```python
from build123d import *

# Parameters (mm, degrees)
F0_W           = 92.075
F0_H           = 12.7
F1_DEPTH       = 46.0375
F2_R           = 16.8275
F3_DEPTH       = 11.1125
F4_D           = 5.5
F5_R           = 35
F5_R_2         = 16.8275
F6_DEPTH       = 25.4
F7_D           = 12.7
F7_CBORE_D     = 12.7
F7_CBORE_DEPTH = 6.35


# Not quite as in the source:
# - a length typed as a fraction of an inch, garbled in the dataset ("3 / 203.2 mm" for 3/8 in), is restored


with BuildPart() as f1:
    # F0 (on Front) → F1 (new body, symmetric)
    with BuildSketch(Plane.XZ):
        with Locations((7.9375, 6.35)):
            Rectangle(F0_W, F0_H)
    extrude(amount=F1_DEPTH, both=True)

    # F2 (on face) → F3 (cut)
    with BuildSketch(Plane.XY.offset(12.7)):
        Circle(F2_R)
    extrude(amount=-F3_DEPTH, mode=Mode.SUBTRACT)

    # F4 (through all)
    with Locations(Plane.XY.offset(12.7)):
        with Locations((0, 22.5), (22.5, 0), (0, -22.5), (-22.5, 0)):
            Hole(F4_D / 2)

    # F5 (on face) → F6 (intersect)
    with BuildSketch(Plane.XY.offset(12.7)):
        Circle(F5_R)
        Circle(F5_R_2, mode=Mode.SUBTRACT)
        Circle(F5_R_2)
    extrude(amount=-F6_DEPTH, mode=Mode.INTERSECT)

    # F7 (through all)
    with Locations(Plane.XY.offset(12.7)):
        with Locations((0, 0)):
            CounterBoreHole(F7_D / 2, F7_CBORE_D / 2, F7_CBORE_DEPTH)


solid = f1.part
```
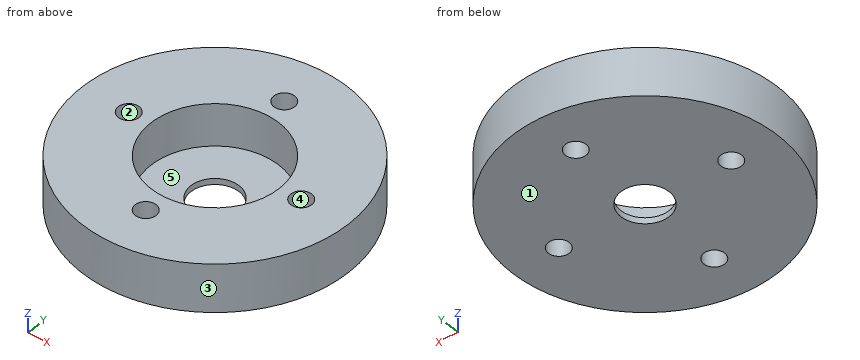
Could you check a few things on this model? Use its own coordinates, in mm. Face numbers are marked on the shaded views. A direction names the side the tool comes from. Round coordinates to 2 decimals unless told otherwise and drop trailing zeros. Write each loop counter-clockwise with the first axis right and the second up, starting at its lowest first coordinate (ties: lowest second). Pieces come first, ordered by that corner, then holes. Notation, with made-up numbers: M 55,25 L 66,25 A23 ccw 66,51 Z; hole C -29.75,34 d1. An arc over 180 degrees is marked long. Answer in a Markdown table with one row per item. Add a question column.
Q1. If I drill on line 1 (Y direction, x = 0, z = 8); line 2 (X direction, y = -2, z = 12.25); line 3 (Y direction, x = -24, z = 3), over which ranges is the centre line in solid material (lowest first)? Write a range as from..to.
Q2. Imagine slicing it at D-D (x = 22.5). Please give me the cut outline in (y, z).
Q3. Imagine slicing it at C-C (z = 4.5). Give the number of separate pieces and of enclosed holes in the cut face, then the cut area to 3 significant figures.
Q4. Will these pins go through, and if not, where does the flat tip stop? pin 1 Ø6 at (x, z) = (-7.5, 6.5) entering from -Y; pin 2 Ø17 at (x, y) = (-3.5, 4) entering from +Z; pin 3 Ø7.5 at (x, y) = (0, 0) entering from +Z; pin 4 Ø6 at (x, z) = (-24.5, 4) entering from -Y.
Q5. If we mould it in two halves opening along Y, with no side actions, what happens to the marked faces 1, 2 and 3? For each: +Y half, -Y half, draft (parallel to the pull), parting line (faces both ways), or undercut.
Q6. On a 3-axis mill with a long thin cutter (end or side, diameter ignored), from which of +Z, -Z, +X, -X, +Y, -Y can I reach the whole of each face in a straight line? I mean the marked faces 4 and 5. Say none if no direction works.
Q7. Imagine slicing it at A-A (x = 0). Please give me the cut outline in (y, z), then the cut area to 3 significant figures.
Values:
| question | item | result |
|---|---|---|
| 1 | line 1 | -35..-25.25, -19.75..-16.83, 16.83..19.75, 25.25..35 |
| 1 | line 2 | -34.94..-24.39, -20.61..-16.71, 16.71..20.61, 24.39..34.94 |
| 1 | line 3 | -25.48..-2.3, 2.3..25.48 |
| 2 | outline | M -26.81,0 L -2.75,0 L -2.75,12.7 L -26.81,12.7 Z; M 2.75,0 L 26.81,0 L 26.81,12.7 L 2.75,12.7 Z |
| 3 | separate pieces | 1 |
| 3 | enclosed holes | 5 |
| 3 | area | 2,860 mm^2 |
| 4 | pin 1 | y = -34.71 |
| 4 | pin 2 | z = 1.59 |
| 4 | pin 3 | through |
| 4 | pin 4 | y = -27.62 |
| 5 | face 1 | draft |
| 5 | face 2 | undercut |
| 5 | face 3 | parting line |
| 6 | face 4 | +Z, -Z |
| 6 | face 5 | +Z |
| 7 | outline | M -35,0 L -25.25,0 L -25.25,12.7 L -35,12.7 Z; M -19.75,0 L -6.35,0 L -6.35,1.59 L -16.83,1.59 L -16.83,12.7 L -19.75,12.7 Z; M 6.35,0 L 19.75,0 L 19.75,12.7 L 16.83,12.7 L 16.83,1.59 L 6.35,1.59 Z; M 25.25,0 L 35,0 L 35,12.7 L 25.25,12.7 Z |
| 7 | area | 355 mm^2 |
